Geometry check sheet. Reference: drawing and pictorial views, mm from the part's lowest x, y, z. A direction names the side the tool comes from. Give positions to 0.01 mm unless a question says otherwise; leave off trailing zeros. Write each loop counter-clockwise with the first axis right and the second up, starting at its lowest first coordinate (ties: lowest second). Pieces come first, ordered by that corner, then holes. Notation, with made-up numbers: (28.5, -25.75) -> (45.5, -25.75) arc R16 cw to (45.5, 1.25) -> close; hole circle Ø1 at (-38.75, 87.25). An arc over 180 degrees is marked (long way). Use a Markdown table: item, result. Add a question column.
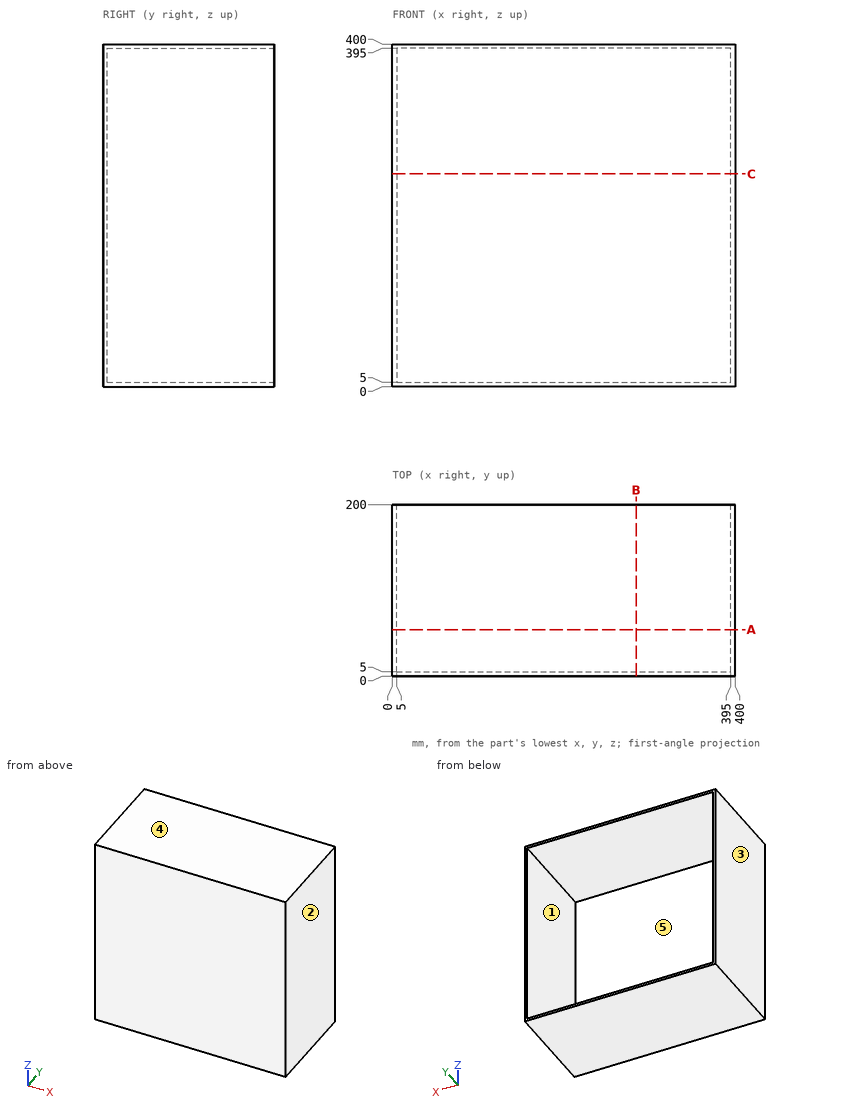
1) Draft check along X on the marked faces 3, 4 and 5. Enter one of: +X half, -X half, draft (parallel to the pull), parting line (faces both ways), or undercut.
2) Sectioned sample at B-B, the plane x = 284.5. Enter the section's corners in (y, z), and give its area (3 significant figures).
3) Sectioned sample at C-C, the plane z = 248.5. Enter the section's corners in (x, y).
4) Tool access check on the marked faces 1 and 2. Record the directions out of +Z, -Z, +X, -X, +Y, -Y that give a thin tool (end or side, any length) a straight path to the whole face; none if there is none.
5) Material ranges on probe 1 along X at (y, z) = (11, 284.5); probe 2 along Y at (x, z) = (236, 137), recorded low to high. Write a range as [from, to].
6) Sectioned sample at A-A, the plane y = 54. Enter the section's corners in (x, z), and give its area (3 significant figures).
7) Gauge pin test, flat end, axial feed: P1, Ø4, axis at x = 235, z = 281.5, coming from the +Y side. Record the tip position at first contact, or that the pin passes through.
Check values:
| question | item | result |
|---|---|---|
| 1 | face 3 | -X half |
| 1 | face 4 | draft |
| 1 | face 5 | undercut |
| 2 | outline | (0, 0) -> (200, 0) -> (200, 5) -> (5, 5) -> (5, 395) -> (200, 395) -> (200, 400) -> (0, 400) -> close |
| 2 | area | 3,950 mm² |
| 3 | outline | (0, 0) -> (400, 0) -> (400, 200) -> (395, 200) -> (395, 5) -> (5, 5) -> (5, 200) -> (0, 200) -> close |
| 4 | face 1 | +Y |
| 4 | face 2 | +Z, -Z, +X, +Y, -Y |
| 5 | probe 1 | [0, 5], [395, 400] |
| 5 | probe 2 | [0, 5] |
| 6 | outline | (0, 0) -> (400, 0) -> (400, 400) -> (0, 400) -> close; hole (5, 5) -> (395, 5) -> (395, 395) -> (5, 395) -> close |
| 6 | area | 7,900 mm² |
| 7 | P1 | y = 5 |
